Verification items for the finished model (mm, model axes). A direction names the side the tool comes from. Give positions to 0.01 mm unless a question says otherwise; leave off trailing zeros. Write each loop counter-clockwise with the first axis right and the second up, starting at its lowest first coordinate (ties: lowest second). Pieces come first, ordered by that corner, then holes. Notation, with made-up numbers: (74, 35) -> (101, 35) arc R19 ccw to (101, 67) -> close; hole circle Ø6 at (34, 55.25). An arc over 180 degrees is marked (long way). Write item = value, one per line.
from build123d import *

# Parameters (mm, degrees)
SKETCH_1_R      = 1.55
SKETCH_1_R_2    = 35
EXTRUDE_1_DEPTH = 3
FILLET_1_R      = 2


with BuildPart() as part:
    # 草图1 → 凸台-拉伸1 (new body)
    with BuildSketch(Plane.XY):
        with BuildLine():
            Line((-4, 0), (-4, 6))
            Line((-4, 6), (16, 6))
            Line((16, 6), (16, 0))
            ThreePointArc((16, 0), (14.487394132, -16.500041247), (10, -32.450045372))
            ThreePointArc((10, -32.450045372), (-34.779762591, -96.755939555), (-19, -20))
            ThreePointArc((-19, -20), (-8.166666667, -12.5), (-4, 0))
        make_face()
        Circle(SKETCH_1_R, mode=Mode.SUBTRACT)
        with Locations((12, 0)):
            Circle(SKETCH_1_R, mode=Mode.SUBTRACT)
        with Locations((-19, -60)):
            Circle(SKETCH_1_R_2, mode=Mode.SUBTRACT)
        with BuildLine():
            Line((1.53004615, -5), (9.8523796, -5))
            ThreePointArc((9.8523796, -5), (8.433483023, -16.219496713), (5.533456158, -27.150197429))
            ThreePointArc((5.533456158, -27.150197429), (-0.758932149, -23.281293002), (-7.64339635, -20.60421909))
            ThreePointArc((-7.64339635, -20.60421909), (-1.701196442, -13.598971308), (1.53004615, -5))
        make_face(mode=Mode.SUBTRACT)
    extrude(amount=EXTRUDE_1_DEPTH)

    # 圆角1
    fillet_1_edges = [part.edges().sort_by_distance(p)[0] for p in [
        (-19, -20, 1.5),
        (10, -32.450045372, 1.5),
        (-7.64339635, -20.60421909, 1.5),
        (5.533456158, -27.150197429, 1.5),
        (9.8523796, -5, 1.5),
        (1.53004615, -5, 1.5),
    ]]
    fillet(fillet_1_edges, radius=FILLET_1_R)


solid = part.part
Item 1: Mould release check, pull along X, two halves, no side actions. Record for faces 1 (the cylindrical face through (-8.19, -12.53, 1.48)), 2 (the cylindrical face through (0.715, -1.375, 1.479)), 3 (the flat face through (-1, -27, 3)): +X half, -X half, draft (parallel to the pull), parting line (faces both ways), or undercut.
Response values:
face_1 = -X half
face_2 = undercut
face_3 = draft
Item 2: Sectioned sample at A-A on x = -38. Record the cut outline in (y, z).
Response values:
outline = (-95.2, 0) -> (-89.39, 0) -> (-89.39, 3) -> (-95.2, 3) -> close; (-30.61, 0) -> (-24.8, 0) -> (-24.8, 3) -> (-30.61, 3) -> close
Item 3: Set-up check for faces 4 (the flat face through (-4, 3, 1)), 5 (the flat face through (5, -5, 1)), 6 (the flat face through (16, 3, 1)): record each of +Z, -Z, +X, -X, +Y, -Y from which the full face is reachable in a straight line by a thin tool's end or side.
Response values:
face_4 = +Z, -Z, -X, +Y
face_5 = +Z, -Z
face_6 = +Z, -Z, +X, +Y
Item 4: Sectioned sample at D-D on z = 1.5. Give the number of separate pieces and of enclosed holes in the cut face, then the cut area to 3 significant figures.
Response values:
separate_pieces = 1
enclosed_holes = 4
area = 1,680 mm^2
Item 5: Sectioned sample at C-C on x = 12. Record the cut outline in (y, z), then the cut area to 3 significant figures.
Response values:
outline = (-85.28, 0) -> (-76.25, 0) -> (-76.25, 3) -> (-85.28, 3) -> close; (-43.75, 0) -> (-34.72, 0) -> (-34.72, 3) -> (-43.75, 3) -> close; (-26.65, 0) -> (-1.55, 0) -> (-1.55, 3) -> (-26.65, 3) -> close; (1.55, 0) -> (6, 0) -> (6, 3) -> (1.55, 3) -> close
area = 143 mm^2
Item 6: Sectioned sample at B-B on y = -69.5. Record the cut outline in (x, z), then the cut area to 3 significant figures.
Response values:
outline = (-57.86, 0) -> (-52.69, 0) -> (-52.69, 3) -> (-57.86, 3) -> close; (14.69, 0) -> (19.86, 0) -> (19.86, 3) -> (14.69, 3) -> close
area = 31.0 mm^2
Item 7: Material ranges on line 1 (Y direction, x = 6, z = 0.5); line 2 (X direction, y = -61.5, z = 2.6); line 3 (Y direction, x = -50.5, z = 0.25), recorded low to high.
Response values:
line_1 = -91.22 to -84.49, -35.51 to -25.23, -5 to 6
line_2 = -58.97 to -53.97, 15.97 to 20.97
line_3 = -84.65 to -75.26, -44.74 to -35.35
